from build123d import *

# Parameters (mm, degrees)
SKETCH_3_R          = 35
EXTRUDE_2_DEPTH     = 74
SKETCH_4_R          = 7.5
SKETCH_4_R_2        = 5
CUT_EXTRUDE_1_DEPTH = 138.830511861


with BuildPart() as part:
    # 草图3 → 凸台-拉伸2 (new body)
    with BuildSketch(Plane.XY):
        with BuildLine():
            Line((-43.5, 0), (43.5, 0))
            Line((43.5, 0), (43.5, 23))
            Line((43.5, 23), (103.5, 23))
            Line((103.5, 23), (103.5, 53))
            Line((103.5, 53), (43.081318457, 53))
            ThreePointArc((43.081318457, 53), (0, 85), (-43.081318457, 53))
            Line((-43.081318457, 53), (-103.5, 53))
            Line((-103.5, 53), (-103.5, 23))
            Line((-103.5, 23), (-43.5, 23))
            Line((-43.5, 23), (-43.5, 0))
        make_face()
        with Locations((0, 40)):
            Circle(SKETCH_3_R, mode=Mode.SUBTRACT)
    extrude(amount=EXTRUDE_2_DEPTH)

    # 草图4 → 切除-拉伸1 (cut, through all)
    with BuildSketch(Plane(origin=(0, 53, 0), x_dir=(1, 0, 0), z_dir=(0, 1, 0))):
        with Locations(Location((86, -17.5, 0), (0, 0, 270))):
            Circle(SKETCH_4_R)
        with Locations(Location((86, -56.5, 0), (0, 0, 270))):
            Circle(SKETCH_4_R)
        with Locations(Location((70.5, -39, 0), (0, 0, 270))):
            Circle(SKETCH_4_R_2)
        with Locations(Location((-86, -17.5, 0), (0, 0, 270))):
            Circle(SKETCH_4_R)
        with Locations(Location((-86, -56.5, 0), (0, 0, 270))):
            Circle(SKETCH_4_R)
        with Locations(Location((-70.5, -39, 0), (0, 0, 270))):
            Circle(SKETCH_4_R_2)
    extrude(amount=-CUT_EXTRUDE_1_DEPTH, mode=Mode.SUBTRACT)


solid = part.part
The listing builds one solid part. Answer for the finished solid, in the listing's coordinates (mm). A direction names the side the tool comes from. Coordinates: 2 decimals unless noted, no trailing zeros. Loops run counter-clockwise (first coordinate to the right, second up) from the corner with the lowest first, then second, coordinate; pieces in that order, holes last.
1) Flat-ended cylindrical pins translate along their axes: pin 1 Ø12 at (x, z) = (-86, 56.5) entering from -Y; pin 2 Ø8 at (x, z) = (-69.5, 30.5) entering from +Y; pin 3 Ø11.5 at (y, z) = (9, 53.5) entering from -X; pin 4 Ø8 at (y, z) = (21, 49) entering from -X. Find the tip coordinate at first contact, or state that the pin passes through.
2) Find section B-B on x = 70.5. Write down the section's boundary in (y, z), then the cut area to 3 significant figures.
3) Determine the mould class of faces 1 (the face through (0.805, 84.993, 36.482)), 2 (the face through (-93.32, 38.21, 15.87)), 3 (the face through (70.72, 38.21, 34.005)), 4 (the face through (-1, 0, 36)) for opening direction X: pulls with the +X half, pulls with the -X half, needs draft (parallel to the pull), parting line crosses it, or undercut.
4) Find the intervals of material crossed by L1, parallel to X at y = 27.5, z = 53; L2, parallel to X at y = 46.25, z = 39; L3, parallel to Y at x = 76, z = 12, in increasing order.
5) Find section C-C on y = 36. Write down the section's boundary in (x, z), then the cut area to 3 significant figures.
6) A tool of negligible diameter and unlimited length cuts with its end or side. For faces 5 (the face through (80, 23, 36)), 6 (the face through (-66, 53, 36)), 7 (the face through (-43.5, 12, 36)), from which of +Z, -Z, +X, -X, +Y, -Y can it reach the whole face along a straight path? Write none if from no direction.
7) Find section D-D on z = 61. Write down the section's boundary in (x, y).
8) Find section A-A on z = 39. Write down the section's boundary in (x, y).
Values:
1. pin 1: passes through
1. pin 2: stops at y = 53
1. pin 3: stops at x = -43.5
1. pin 4: stops at x = -103.5
2. outline: (23, 0) - (53, 0) - (53, 34) - (23, 34) - close; (23, 44) - (53, 44) - (53, 74) - (23, 74) - close
2. area: 1,920 mm2
3. face 1: parting line crosses it
3. face 2: undercut
3. face 3: undercut
3. face 4: needs draft
4. L1: x = -103.5 to -92.63, -79.37 to -32.69, 32.69 to 79.37, 92.63 to 103.5
4. L2: x = -103.5 to -75.5, -65.5 to -34.44, 34.44 to 65.5, 75.5 to 103.5
4. L3: y = 23 to 53
5. outline: (-103.5, 0) - (-34.77, 0) - (-34.77, 74) - (-103.5, 74) - close; (34.77, 0) - (103.5, 0) - (103.5, 74) - (34.77, 74) - close; hole circle Ø15 at (-86, 17.5); hole circle Ø15 at (-86, 56.5); hole circle Ø10 at (-70.5, 39); hole circle Ø10 at (70.5, 39); hole circle Ø15 at (86, 17.5); hole circle Ø15 at (86, 56.5)
5. area: 9,310 mm2
6. face 5: +Z, -Z, +X, -Y
6. face 6: +Z, -Z, -X, +Y
6. face 7: +Z, -Z, -X, -Y
7. outline: (-103.5, 23) - (-92, 23) - (-92, 53) - (-103.5, 53) - close; (-80, 23) - (-43.5, 23) - (-43.5, 0) - (43.5, 0) - (43.5, 23) - (80, 23) - (80, 53) - (43.08, 53) arc R45 ccw to (-43.08, 53) - (-80, 53) - close; (92, 23) - (103.5, 23) - (103.5, 53) - (92, 53) - close; hole circle Ø70 at (0, 40)
8. outline: (-103.5, 23) - (-75.5, 23) - (-75.5, 53) - (-103.5, 53) - close; (-65.5, 23) - (-43.5, 23) - (-43.5, 0) - (43.5, 0) - (43.5, 23) - (65.5, 23) - (65.5, 53) - (43.08, 53) arc R45 ccw to (-43.08, 53) - (-65.5, 53) - close; (75.5, 23) - (103.5, 23) - (103.5, 53) - (75.5, 53) - close; hole circle Ø70 at (0, 40)
